```python
from build123d import *

# Parameters (mm, degrees)
F2_START = 25
F2_DEPTH = 75
F3_DEPTH = 55
F5_DEPTH = 4


with BuildPart() as f2:
    # F1 (on Right) → F2 (new body)
    with BuildSketch(Plane.YZ.offset(F2_START)):
        Polygon((-16.625, 0), (0, 0), (16.625, 0), (16.625, 20), (-16.625, 20), align=None)
    extrude(amount=F2_DEPTH)

    # F0 (on Top) → F3 (join)
    with BuildSketch(Plane.XY):
        with BuildLine():
            ThreePointArc((33.25, 36.25), (40.6239406019, 35.4920765806), (47.6895290782, 33.25))
            Line((47.6895290782, 33.25), (89.3104709218, 33.25))
            ThreePointArc((89.3104709218, 33.25), (96.3760593981, 35.4920765806), (103.75, 36.25))
            Line((103.75, 36.25), (33.25, 36.25))
        make_face()
        with BuildLine():
            ThreePointArc((65.4629147238, 16.625), (58.0130830961, 26.4736135723), (47.6895290782, 33.25))
            ThreePointArc((47.6895290782, 33.25), (40.6239406019, 35.4920765806), (33.25, 36.25))
            ThreePointArc((33.25, 36.25), (-3, 0), (33.25, -36.25))
            ThreePointArc((33.25, -36.25), (40.6239406019, -35.4920765806), (47.6895290782, -33.25))
            ThreePointArc((47.6895290782, -33.25), (58.0130830961, -26.4736135723), (65.4629147238, -16.625))
            Line((65.4629147238, -16.625), (71.5370852762, -16.625))
            ThreePointArc((71.5370852762, -16.625), (78.9869169039, -26.4736135723), (89.3104709218, -33.25))
            ThreePointArc((89.3104709218, -33.25), (96.3760593981, -35.4920765806), (103.75, -36.25))
            ThreePointArc((103.75, -36.25), (140, 0), (103.75, 36.25))
            ThreePointArc((103.75, 36.25), (96.3760593981, 35.4920765806), (89.3104709218, 33.25))
            ThreePointArc((89.3104709218, 33.25), (78.9869169039, 26.4736135723), (71.5370852762, 16.625))
            Line((71.5370852762, 16.625), (65.4629147238, 16.625))
        make_face()
        with BuildLine():
            ThreePointArc((33.25, -33.25), (0, 0), (33.25, 33.25))
            ThreePointArc((33.25, 33.25), (56.7613004745, 23.5113004745), (66.5, 0))
            ThreePointArc((66.5, 0), (56.7613004745, -23.5113004745), (33.25, -33.25))
        make_face(mode=Mode.SUBTRACT)
        with BuildLine():
            ThreePointArc((137, 0), (127.2613004745, -23.5113004745), (103.75, -33.25))
            ThreePointArc((103.75, -33.25), (70.5, 0), (103.75, 33.25))
            ThreePointArc((103.75, 33.25), (127.2613004745, 23.5113004745), (137, 0))
        make_face(mode=Mode.SUBTRACT)
        with BuildLine():
            ThreePointArc((47.6895290782, -33.25), (40.6239406019, -35.4920765806), (33.25, -36.25))
            Line((33.25, -36.25), (103.75, -36.25))
            ThreePointArc((103.75, -36.25), (96.3760593981, -35.4920765806), (89.3104709218, -33.25))
            Line((89.3104709218, -33.25), (47.6895290782, -33.25))
        make_face()
    extrude(amount=F3_DEPTH)

    # F4 (on face) → F5 (join)
    with BuildSketch(Plane(origin=(0, 0, 0), x_dir=(1, 0, 0), z_dir=(0, 0, -1))):
        with BuildLine():
            Line((103.75, 36.25), (33.25, 36.25))
            ThreePointArc((33.25, 36.25), (7.6173792195, 25.6326208556), (-3, 1.062e-07))
            ThreePointArc((-3, 1.062e-07), (6.493803342, -24.4574822989), (30.0023968175, -36.1042320728))
            Line((30.0023968175, -36.1042320728), (106.9976031825, -36.1042320728))
            ThreePointArc((106.9976031825, -36.1042320728), (139.9635396823, 1.6254364583), (103.75, 36.25))
        make_face()
        with BuildLine():
            ThreePointArc((47.6895290782, -33.25), (58.0130830961, -26.4736135723), (65.4629147238, -16.625))
            Line((65.4629147238, -16.625), (71.5370852762, -16.625))
            ThreePointArc((71.5370852762, -16.625), (78.9869169039, -26.4736135723), (89.3104709218, -33.25))
            Line((89.3104709218, -33.25), (47.6895290782, -33.25))
        make_face(mode=Mode.SUBTRACT)
        with BuildLine():
            Line((100, 16.625), (74.9546553242, 16.625))
            ThreePointArc((74.9546553242, 16.625), (132.5453446758, 16.625), (103.75, -33.25))
            ThreePointArc((103.75, -33.25), (87.125, -28.7953446758), (74.9546553242, -16.625))
            Line((74.9546553242, -16.625), (100, -16.625))
            Line((100, -16.625), (100, 16.625))
        make_face(mode=Mode.SUBTRACT)
        with BuildLine():
            Line((25, -16.625), (62.0453446758, -16.625))
            ThreePointArc((62.0453446758, -16.625), (4.4546553242, -16.625), (33.25, 33.25))
            ThreePointArc((33.25, 33.25), (49.875, 28.7953446758), (62.0453446758, 16.625))
            Line((62.0453446758, 16.625), (25, 16.625))
            Line((25, 16.625), (25, -16.625))
        make_face(mode=Mode.SUBTRACT)
        with BuildLine():
            ThreePointArc((89.3104709218, 33.25), (78.9869169039, 26.4736135723), (71.5370852762, 16.625))
            Line((71.5370852762, 16.625), (65.4629147238, 16.625))
            ThreePointArc((65.4629147238, 16.625), (58.0130830961, 26.4736135723), (47.6895290782, 33.25))
            Line((47.6895290782, 33.25), (89.3104709218, 33.25))
        make_face(mode=Mode.SUBTRACT)
        with BuildLine():
            Line((33.25, 36.25), (-3, 36.25))
            Line((-3, 36.25), (-3, 1.062e-07))
            ThreePointArc((-3, 1.062e-07), (7.6173792195, 25.6326208556), (33.25, 36.25))
        make_face()
        with BuildLine():
            Line((140.309497714, 36.25), (103.75, 36.25))
            ThreePointArc((103.75, 36.25), (139.9635396823, 1.6254364583), (106.9976031825, -36.1042320728))
            Line((106.9976031825, -36.1042320728), (140.309497714, -36.1042320728))
            Line((140.309497714, -36.1042320728), (140.309497714, 36.25))
        make_face()
        with BuildLine():
            Line((65.4629147238, 16.625), (71.5370852762, 16.625))
            ThreePointArc((71.5370852762, 16.625), (78.9869169039, 26.4736135723), (89.3104709218, 33.25))
            Line((89.3104709218, 33.25), (47.6895290782, 33.25))
            ThreePointArc((47.6895290782, 33.25), (58.0130830961, 26.4736135723), (65.4629147238, 16.625))
        make_face()
        with BuildLine():
            ThreePointArc((33.25, 33.25), (4.4546553242, -16.625), (62.0453446758, -16.625))
            Line((62.0453446758, -16.625), (25, -16.625))
            Line((25, -16.625), (25, 16.625))
            Line((25, 16.625), (62.0453446758, 16.625))
            ThreePointArc((62.0453446758, 16.625), (49.875, 28.7953446758), (33.25, 33.25))
        make_face()
        with BuildLine():
            ThreePointArc((103.75, -33.25), (132.5453446758, 16.625), (74.9546553242, 16.625))
            Line((74.9546553242, 16.625), (100, 16.625))
            Line((100, 16.625), (100, -16.625))
            Line((100, -16.625), (74.9546553242, -16.625))
            ThreePointArc((74.9546553242, -16.625), (87.125, -28.7953446758), (103.75, -33.25))
        make_face()
        with BuildLine():
            Line((71.5370852762, -16.625), (65.4629147238, -16.625))
            ThreePointArc((65.4629147238, -16.625), (58.0130830961, -26.4736135723), (47.6895290782, -33.25))
            Line((47.6895290782, -33.25), (89.3104709218, -33.25))
            ThreePointArc((89.3104709218, -33.25), (78.9869169039, -26.4736135723), (71.5370852762, -16.625))
        make_face()
        with BuildLine():
            ThreePointArc((30.0023968175, -36.1042320728), (6.493803342, -24.4574822989), (-3, 1.062e-07))
            Line((-3, 1.062e-07), (-3, -36.1042320728))
            Line((-3, -36.1042320728), (30.0023968175, -36.1042320728))
        make_face()
    extrude(amount=F5_DEPTH)


solid = f2.part
```
Geometry check sheet. Reference: the model listing, model coordinates, mm. A direction names the side the tool comes from. Give positions to 0.01 mm unless a question says otherwise; leave off trailing zeros. Order: outer loops, then holes, each group sorted by start corner. A loop starts at its lowest first (then second) coordinate and runs counter-clockwise, first axis right, second up. Notation, with made-up numbers: (-33, 84.5) - (-17, 84.5) arc R22 cw to (-17, 101.5) - close; hole circle Ø8 at (27.25, -2.75). An arc over 180 degrees is marked (long way). Write item = value, one per line. Start each with the question number.
1) Access from +Z, -Z, +X, -X, +Y, -Y to the whole of each face (thin tool, end or side, straight path). Record for faces 1 (the flat face through (69, 16.625, 27)), 2 (the cylindrical face through (139.99, -0.8, 27.12)), 3 (the flat face through (68, 36.104, -2)).
2) Gauge pin test, flat ends, axial feed: pin 1 Ø5 at (x, y) = (36.5, 11.5) entering from +Z; pin 2 Ø8.5 at (x, y) = (68, -27.5) entering from +Z; pin 3 Ø12 at (y, z) = (-14, 23) entering from +X. Record the tip position at first contact, or that the pin passes through.
3) Section check A-A (z = 13.5). Enter the section's corners in (x, y) (3 decimals), then the cut area to 3 significant figures.
4) Scan lines: L1, parallel to Y at x = 67.5, z = 14 (3 decimals); L2, parallel to X at y = -20, z = 21; L3, parallel to X at y = -12, z = 1. Record each from-to range of solid material in increasing order.
5) Section check C-C (y = 25.5). Enter the section's corners in (x, z).
6) Draft check along X on faces 4 (the flat face through (68, 0, 55)), 5 (the flat face through (87, -16.625, 10)), 6 (the cylindrical face through (-2.99, 0.8, 27.12)). Enter one of: released by +X, released by -X, zero draft, split by the parting line, or undercut.
7) Section check D-D (z = 38.5). Enter the section's corners in (x, y) (3 decimals), then the cut area to 3 significant figures.
8) Section check B-B (x = 18). Enter the section's corners in (y, z), then the cut area to 3 significant figures.
Geometry check:
q1.face_1 = +Z
q1.face_2 = +Z, +X
q1.face_3 = -Z, +X, -X, +Y
q2.pin_1 = 20
q2.pin_2 = 0
q2.pin_3 = 139.11
q3.outline = (33.25, -36.25) - (103.75, -36.25) arc R36.25 ccw to (103.75, 36.25) - (33.25, 36.25) arc R36.25 ccw to start; hole (25, -16.625) - (25, 16.625) - (62.045, 16.625) arc R33.25 ccw (long way) to (62.045, -16.625) - close; hole (47.69, -33.25) - (89.31, -33.25) arc R36.25 cw to (71.537, -16.625) - (65.463, -16.625) arc R36.25 cw to start; hole (47.69, 33.25) arc R36.25 cw to (65.463, 16.625) - (71.537, 16.625) arc R36.25 cw to (89.31, 33.25) - close; hole (74.955, -16.625) arc R33.25 ccw (long way) to (74.955, 16.625) - (100, 16.625) - (100, -16.625) - close
q3.area = 3,900 mm2
q4.L1 = -36.25 to -33.25, -16.625 to 16.625, 33.25 to 36.25
q4.L2 = 3.02 to 6.69, 59.81 to 63.48, 73.52 to 77.19, 130.31 to 133.98
q4.L3 = -0.96 to 2.24, 25 to 100, 134.76 to 137.96
q5.outline = (-3, -4) - (140.31, -4) - (140.31, 0) - (129.51, 0) - (129.51, 55) - (125.09, 55) - (125.09, 0) - (82.41, 0) - (82.41, 55) - (77.99, 55) - (77.99, 0) - (59.01, 0) - (59.01, 55) - (54.59, 55) - (54.59, 0) - (11.91, 0) - (11.91, 55) - (7.49, 55) - (7.49, 0) - (-3, 0) - close
q6.face_4 = zero draft
q6.face_5 = undercut
q6.face_6 = released by -X
q7.outline = (33.25, -36.25) - (103.75, -36.25) arc R36.25 ccw to (103.75, 36.25) - (33.25, 36.25) arc R36.25 ccw to start; hole circle Ø66.5 at (33.25, 0); hole (47.69, -33.25) - (89.31, -33.25) arc R36.25 cw to (71.537, -16.625) - (65.463, -16.625) arc R36.25 cw to start; hole (47.69, 33.25) arc R36.25 cw to (65.463, 16.625) - (71.537, 16.625) arc R36.25 cw to (89.31, 33.25) - close; hole circle Ø66.5 at (103.75, 0)
q7.area = 1,640 mm2
q8.outline = (-36.25, -4) - (36.1, -4) - (36.1, 0) - (32.89, 0) - (32.89, 55) - (29.55, 55) - (29.55, 0) - (-29.55, 0) - (-29.55, 55) - (-32.89, 55) - (-32.89, 0) - (-36.25, 0) - close
q8.area = 657 mm2
